The model under review builds one solid part; all positions refer to its coordinate system, in mm. A direction names the side the tool comes from. Round coordinates to 2 decimals unless told otherwise and drop trailing zeros. Write each loop counter-clockwise with the first axis right and the second up, starting at its lowest first coordinate (ties: lowest second). Pieces come first, ordered by that corner, then holes. Notation, with made-up numbers: (63, 38.25) -> (70, 38.25) arc R19 ccw to (70, 71.25) -> close; hole circle Ø11 at (-0.75, 65.25). An arc over 180 degrees is marked (long way). Return JSON: item names as keys, results as strings. Group by question number.
1. Take a section at C-C, the plane z = 11.5. Write out the cut boundary in (x, y), then the cut area to 3 significant figures.
2. Take a section at A-A, the plane x = -45. Write out the cut boundary in (y, z).
3. Take a section at D-D, the plane x = -30. Write out the cut boundary in (y, z).
4. Tool access review of faces 1 (the flat face through (-68.93, -12.52, 9.31)), 2 (the cylindrical face through (15.36, -12.52, -1.37)), 3 (the flat face through (-8, -25.4, 16)), 4 (the cylindrical face through (-57.17, -12.52, -1.18)), 5 (the flat face through (-27.01, -12.52, 11.26)): name each direction out of +Z, -Z, +X, -X, +Y, -Y from which nothing blocks a thin tool from reaching the whole face with its end or side.
5. Take a section at B-B, the plane y = -14.5. Write out the cut boundary in (x, z), then the cut area to 3 significant figures.
6. For line 1 along Z through (x, y) = (-32, -4.25); line 2 along X through (y, z) = (-7.5, 28); line 3 along Z through (x, y) = (-12.5, -15.25), list the stretches that pass through material, from the lowest coordinate up. Write a range as from..to.
7. Mouldability with a two-part tool opening along Z and no side actions: class faces 6 (the flat face through (28.743, -12.522, 19.583)), 7 (the flat face through (27.953, -12.522, 9.206)), 8 (the cylindrical face through (8.278, -12.522, -26.498)) as pulls with the +Z half, pulls with the -Z half, needs draft (parallel to the pull), parting line crosses it, or undercut.
8. Clearance check with flat-ended pins moving along their axes: P1, Ø5, axis at y = -6, z = 42.5, coming from the -X side; P2, Ø5, axis at x = -42, z = 27.5, coming from the -Y side; P3, Ø10, axis at x = -30.5, y = -21, coming from the -Z side; P4, Ø3, axis at y = -22.5, z = -5, coming from the +X side. State where each tip first meets the part, or that it passes through.
from build123d import *

# Parameters (mm, degrees)
F0_R     = 11.591064
F0_R_2   = 8.286471
F1_DEPTH = 25.4


with BuildPart() as f1:
    # F0 (on Front) → F1 (new body)
    with BuildSketch(Plane.XZ):
        with BuildLine():
            ThreePointArc((18.303812, 5.605529), (19.740788, 11.737184), (20.223563, 18.016437))
            ThreePointArc((20.223563, 18.016437), (20.00443, 22.253734), (19.349371, 26.445823))
            ThreePointArc((19.349371, 26.445823), (-20.85367, 59.09367), (-61.056712, 26.445823))
            ThreePointArc((-61.056712, 26.445823), (-61.879304, 15.958178), (-60.011153, 5.605529))
            ThreePointArc((-60.011153, 5.605529), (-57.118422, -1.276225), (-53.028005, -7.520816))
            ThreePointArc((-53.028005, -7.520816), (-43.541093, -16.227101), (-31.824876, -21.568556))
            ThreePointArc((-31.824876, -21.568556), (-20.85367, -23.060796), (-9.882464, -21.568556))
            ThreePointArc((-9.882464, -21.568556), (1.833753, -16.227101), (11.320664, -7.520816))
            ThreePointArc((11.320664, -7.520816), (15.411082, -1.276225), (18.303812, 5.605529))
        make_face()
        Polygon((-33.3375, 18.016437), (-20.85367, 18.016437), (-11.490798, 18.016437), (-20.85367, 4.681436), align=None, mode=Mode.SUBTRACT)
        with Locations((-36.742181, 33.053778)):
            Circle(F0_R, mode=Mode.SUBTRACT)
        with Locations((-6.951223, 31.351436)):
            Circle(F0_R_2, mode=Mode.SUBTRACT)
        with BuildLine():
            ThreePointArc((19.349371, 26.445823), (20.00443, 22.253734), (20.223563, 18.016437))
            ThreePointArc((20.223563, 18.016437), (19.740788, 11.737184), (18.303812, 5.605529))
            Line((18.303812, 5.605529), (37.877075, 12.909415))
            Line((37.877075, 12.909415), (19.349371, 26.445823))
        make_face()
        with BuildLine():
            ThreePointArc((-60.011153, 5.605529), (-61.879304, 15.958178), (-61.056712, 26.445823))
            Line((-61.056712, 26.445823), (-77.598356, 12.909415))
            Line((-77.598356, 12.909415), (-60.011153, 5.605529))
        make_face()
        with BuildLine():
            ThreePointArc((-9.882464, -21.568556), (8.530379, -26.334736), (11.320664, -7.520816))
            ThreePointArc((11.320664, -7.520816), (1.833753, -16.227101), (-9.882464, -21.568556))
        make_face()
        with BuildLine():
            ThreePointArc((-31.824876, -21.568556), (-43.541093, -16.227101), (-53.028005, -7.520816))
            ThreePointArc((-53.028005, -7.520816), (-50.003519, -25.981242), (-31.824876, -21.568556))
        make_face()
    extrude(amount=F1_DEPTH)


solid = f1.part
Output:
{
 "1": {"outline": "(-74.2, -25.4) -> (-27.24, -25.4) -> (-27.24, 0) -> (-74.2, 0) -> close; (-16.07, -25.4) -> (34.1, -25.4) -> (34.1, 0) -> (-16.07, 0) -> close", "area": "2,470 mm^2"},
 "2": {"outline": "(-25.4, -27.94) -> (0, -27.94) -> (0, 24.92) -> (-25.4, 24.92) -> close; (-25.4, 41.19) -> (0, 41.19) -> (0, 51.25) -> (-25.4, 51.25) -> close"},
 "3": {"outline": "(-25.4, -22.03) -> (0, -22.03) -> (0, 14.45) -> (-25.4, 14.45) -> close; (-25.4, 18.02) -> (0, 18.02) -> (0, 23.63) -> (-25.4, 23.63) -> close; (-25.4, 42.48) -> (0, 42.48) -> (0, 58.06) -> (-25.4, 58.06) -> close"},
 "4": {"face 1": "-Z, -X, +Y, -Y", "face 2": "+X, +Y, -Y", "face 3": "+Z, -Z, +X, -X, -Y", "face 4": "-X, +Y, -Y", "face 5": "+Y, -Y"},
 "5": {"outline": "(-77.6, 12.91) -> (-60.01, 5.61) arc R41.08 ccw to (-53.03, -7.52) arc R12.75 ccw (long way) to (-31.82, -21.57) arc R41.08 ccw to (-9.88, -21.57) arc R12.79 ccw (long way) to (11.32, -7.52) arc R41.08 ccw to (18.3, 5.61) -> (37.88, 12.91) -> (19.35, 26.45) arc R41.08 ccw to (-61.06, 26.45) -> close; hole circle Ø23.18 at (-36.74, 33.05); hole (-33.34, 18.02) -> (-20.85, 4.68) -> (-11.49, 18.02) -> close; hole circle Ø16.57 at (-6.95, 31.35)", "area": "5,360 mm^2"},
 "6": {"line 1": "z = -21.87..16.59, 18.02..22.48, 43.63..57.55", "line 2": "x = -60.7..-47.17, -26.31..-14.53, 0.63..18.99", "line 3": "z = -22.2..16.58, 18.02..25.2, 37.51..58.24"},
 "7": {"face 6": "pulls with the +Z half", "face 7": "pulls with the -Z half", "face 8": "undercut"},
 "8": {"P1": "stops at x = -55.55", "P2": "passes through", "P3": "stops at z = -25.69", "P4": "stops at x = 14.14"}
}
